from build123d import *

# Parameters (mm, degrees)
F1_DEPTH = 19.05
F2_SIZE  = 9.52499


# Not quite as in the source:
# - a fillet or chamfer is up to 0.001 mm smaller than in the source, because OpenCascade refuses the exact size


with BuildPart() as f1:
    # F0 (on Front) → F1 (new body)
    with BuildSketch(Plane.XZ):
        with BuildLine():
            Line((301.9656721215, 276.6333943507), (-155.2343278785, 276.6333943507))
            Line((-155.2343278785, 276.6333943507), (-155.2343278785, 16.2833943507))
            ThreePointArc((-155.2343278785, 16.2833943507), (-141.7639436969, 10.7037785323), (-136.1843278785, -2.7666056493))
            Line((-136.1843278785, -2.7666056493), (-136.1843278785, -161.5166056493))
            Line((-136.1843278785, -161.5166056493), (244.8156721215, -161.5166056493))
            ThreePointArc((244.8156721215, -161.5166056493), (252.4723202952, -132.9416056493), (273.3906721215, -112.023253823))
            ThreePointArc((273.3906721215, -112.023253823), (294.3090239478, -91.1049019968), (301.9656721215, -62.5299019968))
            Line((301.9656721215, -62.5299019968), (301.9656721215, 276.6333943507))
        make_face()
    extrude(amount=-F1_DEPTH)

    # F2 (size 9.525 in the source; OpenCascade refuses exactly that, so slightly less here)
    f2_edges = [f1.edges().sort_by_distance(p)[0] for p in [
        (-155.234328, 0, 146.458394),
        (-155.234328, 19.05, 146.458394),
    ]]
    chamfer(f2_edges, length=F2_SIZE)


solid = f1.part
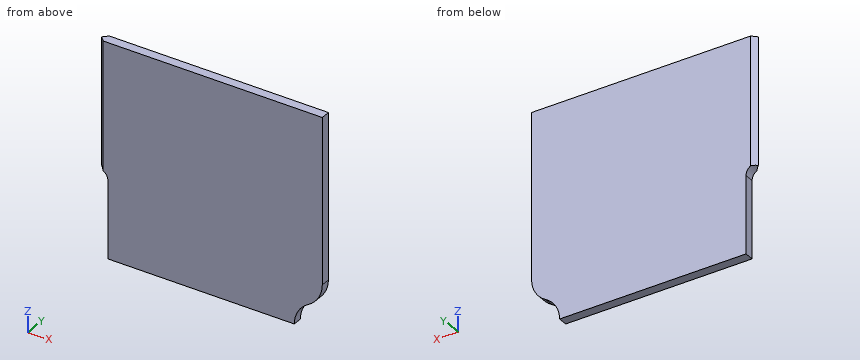
Build history of the part. All positions in model axes, mm. Round coordinates to 2 decimals unless told otherwise and drop trailing zeros. Write each loop counter-clockwise with the first axis right and the second up, starting at its lowest first coordinate (ties: lowest second). Pieces come first, ordered by that corner, then holes. Notation, with made-up numbers: (73, -18) - (125, -18) arc R28 cw to (125, 7) - close; hole circle Ø7 at (50, -21). An arc over 180 degrees is marked (long way). One line per question, with ' | ' between items.
1. Band-saw the part on A-A, the plane z = -40. Write the cut outline in (x, y).
Results are:
outline: (-136.18, 0) - (301.97, 0) - (301.97, 19.05) - (-136.18, 19.05) - close
2. Band-saw the part on B-B, the plane x = 264.5. Write the cut outline in (y, z), and give its area (3 significant figures).
Results are:
outline: (0, -118.36) - (19.05, -118.36) - (19.05, 276.63) - (0, 276.63) - close | area: 7,520 mm^2
3. Drill centre lines: line 1 along X through (y, z) = (7.5, -11); line 2 along Z through (x, y) = (283, 13.5); line 3 along Z through (x, y) = (255, 3.75). Where is each one in solid material? Low to high. Write a range as from..to.
Results are:
line 1: -136.18..301.97 | line 2: -105.05..276.63 | line 3: -128.95..276.63
4. Drop a flat-ended pin along its axis: pin 1 Ø3 at (y, z) = (6, -6.5) entering from -X. Give the stop position or say it passes through.
Results are:
pin 1: x = -136.18
